Part model, mm, in its own coordinate system. Face numbers are marked on the shaded views. Give positions to 0.01 mm unless a question says otherwise; leave off trailing zeros. Order: outer loops, then holes, each group sorted by start corner. A loop starts at its lowest first (then second) coordinate and runs counter-clockwise, first axis right, second up. Notation, with made-up numbers: (63.5, 17) - (113.5, 17) arc R21 cw to (113.5, 45) - close; hole circle Ø8 at (31.5, 40). An arc over 180 degrees is marked (long way). One line per item, written item: value.
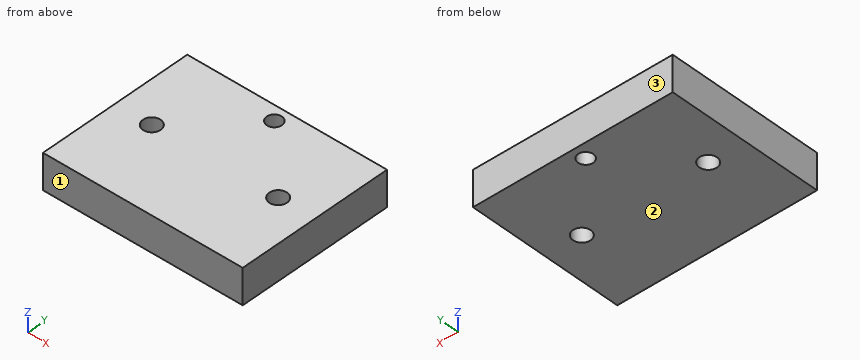
```python
from build123d import *

# Parameters (mm, degrees)
F0_W     = 79
F0_H     = 62
F2_DEPTH = 14
F1_R     = 3.5
F1_R_2   = 3
F3_DEPTH = 14.001


with BuildPart() as f2:
    # F0 (on Top) → F2 (new body)
    with BuildSketch(Plane.XY):
        with Locations((39.5, 31)):
            Rectangle(F0_W, F0_H)
    extrude(amount=-F2_DEPTH)

    # F1 (on face) → F3 (cut, through all)
    with BuildSketch(Plane.XY):
        with Locations((14.5, 31)):
            Circle(F1_R)
        with Locations((39.5, 56.5)):
            Circle(F1_R_2)
        with Locations((64.5, 31)):
            Circle(F1_R)
    extrude(amount=-F3_DEPTH, mode=Mode.SUBTRACT)


solid = f2.part
```
1) Wall check: line 1 along Y through (x, z) = (14.5, -4.75); line 2 along Y through (x, z) = (39.5, -3.5); line 3 along X through (y, z) = (55.5, -6). Give the ranges that are in metal, low to high. Write a range as [from, to].
Answer:
line 1: y = [0, 27.5], [34.5, 62]
line 2: y = [0, 53.5], [59.5, 62]
line 3: x = [0, 36.67], [42.33, 79]
2) Two-plate mould, pull along Y, no slides. Class the marked faces 1, 2 and 3: pulls with the +Y half, pulls with the -Y half, needs draft (parallel to the pull), parting line crosses it, or undercut.
Answer:
face 1: pulls with the -Y half
face 2: needs draft
face 3: pulls with the +Y half
3) Slice it at A-A on y = 31. Write the cut outline in (x, z), then the cut area to 3 significant figures.
Answer:
outline: (0, -14) - (11, -14) - (11, 0) - (0, 0) - close; (18, -14) - (61, -14) - (61, 0) - (18, 0) - close; (68, -14) - (79, -14) - (79, 0) - (68, 0) - close
area: 910 mm2
4) Slice it at C-C on y = 56.5. Write the cut outline in (x, z), then the cut area to 3 significant figures.
Answer:
outline: (0, -14) - (36.5, -14) - (36.5, 0) - (0, 0) - close; (42.5, -14) - (79, -14) - (79, 0) - (42.5, 0) - close
area: 1,020 mm2
5) Slice it at D-D on z = -10.75. Write the cut outline in (x, y), then the cut area to 3 significant figures.
Answer:
outline: (0, 0) - (79, 0) - (79, 62) - (0, 62) - close; hole circle Ø7 at (14.5, 31); hole circle Ø6 at (39.5, 56.5); hole circle Ø7 at (64.5, 31)
area: 4,790 mm2
6) Slice it at B-B on x = 14.5. Write the cut outline in (y, z), then the cut area to 3 significant figures.
Answer:
outline: (0, -14) - (27.5, -14) - (27.5, 0) - (0, 0) - close; (34.5, -14) - (62, -14) - (62, 0) - (34.5, 0) - close
area: 770 mm2
7) Drop a flat-ended pin along its axis: P1, Ø8, axis at x = 64.5, y = 31, coming from the +Z side. Give the stop position or say it passes through.
Answer:
P1: stops at z = 0
